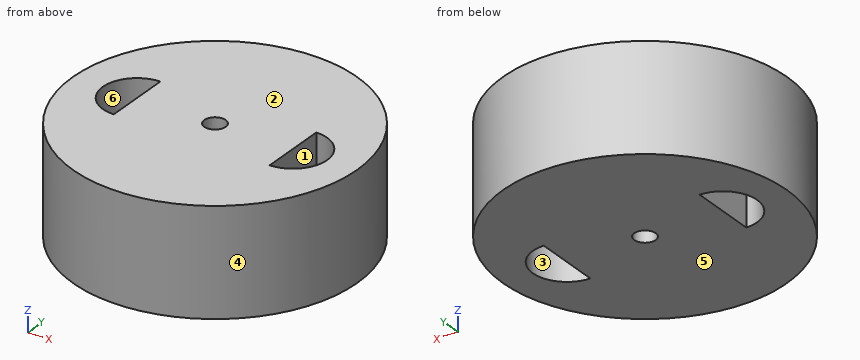
```python
from build123d import *

# Parameters (mm, degrees)
SKETCH1_R               = 101.6
BOSS_EXTRUDE1_DEPTH     = 76.2
CUT_EXTRUDE7_DEPTH      = 163.639355631
CUT_EXTRUDE7_DEPTH_BACK = 163.639355631
SKETCH3_R               = 7.62
CUT_EXTRUDE8_DEPTH      = 163.639355631


with BuildPart() as part:
    # Sketch1 → Boss-Extrude1 (new body)
    with BuildSketch(Plane.XY):
        with Locations(Location((0, 0, 0), (0, 0, 180))):
            Circle(SKETCH1_R)
    extrude(amount=BOSS_EXTRUDE1_DEPTH)

    # Sketch2 → Cut-Extrude7 (cut, two sides: drawn at the far end of the back side and taken through both)
    with BuildSketch(Plane.XY.offset(76.2).offset(-CUT_EXTRUDE7_DEPTH_BACK)):
        with BuildLine():
            ThreePointArc((-55.703026842, -24.462175809), (-80.165202651, 0), (-55.703026842, 24.462175809))
            Line((-55.703026842, 24.462175809), (-55.703026842, -24.462175809))
        make_face()
        with BuildLine():
            Line((55.703026842, 24.462175809), (55.703026842, -24.462175809))
            ThreePointArc((55.703026842, -24.462175809), (80.165202651, 0), (55.703026842, 24.462175809))
        make_face()
    extrude(amount=CUT_EXTRUDE7_DEPTH + CUT_EXTRUDE7_DEPTH_BACK, mode=Mode.SUBTRACT)

    # Sketch3 → Cut-Extrude8 (cut, through all)
    with BuildSketch(Plane.XY.offset(76.2)):
        Circle(SKETCH3_R)
    extrude(amount=-CUT_EXTRUDE8_DEPTH, mode=Mode.SUBTRACT)


solid = part.part
```
For this review, take the finished solid that the model builds, in its own axes (mm). Face numbers are marked on the shaded views. A direction names the side the tool comes from. Round coordinates to 2 decimals unless told otherwise and drop trailing zeros. Write each loop counter-clockwise with the first axis right and the second up, starting at its lowest first coordinate (ties: lowest second). Pieces come first, ordered by that corner, then holes. Notation, with made-up numbers: (82.5, 88.5) - (93.5, 88.5) arc R29 ccw to (93.5, 119.5) - close; hole circle Ø1 at (57.5, -36.75). An arc over 180 degrees is marked (long way). Answer as CSV lines item,"result". Start each with the question number.
(1) For line 1 (Y direction, x = 0, z = 17.5); line 2 (X direction, y = -16.5, z = 48.5); line 3 (X direction, y = -19, z = 60), list the stretches that pass through material, from the lowest coordinate up.
(2) Machinability: for the marked faces 1 and 2, which of the approach directions +Z, -Z, +X, -X, +Y, -Y give a long, thin tool a straight path to every point of the face, cutting with its end or side? Answer none if there is none.
(3) Add section A-A, the plane x = 0. State the section outline as (y, z) points, plus the area to 3 significant figures.
(4) Add section B-B, the plane y = 0. State the section outline as (x, z) points, plus the area to 3 significant figures.
(5) For pin 1 (5 mm diameter, centred on x = 10, z = 27, fed in from -Y); pin 2 (3 mm diameter, centred on x = -45.5, z = 21, fed in from +Y); pin 3 (1.5 mm diameter, centred on y = 16.5, z = 25, fed in from -X), all flat-tipped, find the tip position at first contact; note any pin that passes through.
(6) Mouldability with a two-part tool opening along Y and no side actions: class the marked faces 3, 4, 5 and 6 as +Y half, -Y half, draft (parallel to the pull), parting line (faces both ways), or undercut.
(7) Add section D-D, the plane x = -40.5. State the section outline as (y, z) points.
(8) Add section C-C, the plane z = 8.5. State the section outline as (x, y) points, plus the area to 3 significant figures.
From the geometry:
1,line 1,"y = -101.6 to -7.62, 7.62 to 101.6"
1,line 2,"x = -100.25 to -73.76, -55.7 to 55.7, 73.76 to 100.25"
1,line 3,"x = -99.81 to -71.11, -55.7 to 55.7, 71.11 to 99.81"
2,face 1,"+Z, -Z"
2,face 2,"+Z, +X, -X, +Y, -Y"
3,outline,"(-101.6, 0) - (-7.62, 0) - (-7.62, 76.2) - (-101.6, 76.2) - close; (7.62, 0) - (101.6, 0) - (101.6, 76.2) - (7.62, 76.2) - close"
3,area,"14,300 mm²"
4,outline,"(-101.6, 0) - (-80.17, 0) - (-80.17, 76.2) - (-101.6, 76.2) - close; (-55.7, 0) - (-7.62, 0) - (-7.62, 76.2) - (-55.7, 76.2) - close; (7.62, 0) - (55.7, 0) - (55.7, 76.2) - (7.62, 76.2) - close; (80.17, 0) - (101.6, 0) - (101.6, 76.2) - (80.17, 76.2) - close"
4,area,"10,600 mm²"
5,pin 1,"stops at y = -101.32"
5,pin 2,"stops at y = 91.58"
5,pin 3,"stops at x = -100.37"
6,face 3,"undercut"
6,face 4,"parting line"
6,face 5,"draft"
6,face 6,"undercut"
7,outline,"(-93.18, 0) - (93.18, 0) - (93.18, 76.2) - (-93.18, 76.2) - close"
8,outline,"circle Ø203.2 at (0, 0); hole (-55.7, -24.46) - (-55.7, 24.46) arc R24.46 ccw to start; hole circle Ø15.24 at (0, 0); hole (55.7, -24.46) arc R24.46 ccw to (55.7, 24.46) - close"
8,area,"30,400 mm²"
